from build123d import *

# Parameters (mm, degrees)
F1_DEPTH = 500
F2_R     = 33.415616


with BuildPart() as f1:
    # F0 (on Front) → F1 (new body, symmetric)
    with BuildSketch(Plane.XZ):
        Polygon((-141.84029, 131.140749), (-11.84029, 98.816335), (-11.84029, -98.816335), (-141.84029, -131.140749), (-141.84029, -249.530149), (236.54911, -249.530149), (236.54911, -131.140749), (106.54911, -98.816335), (106.54911, 98.816335), (236.54911, 131.140749), (236.54911, 249.530149), (-141.84029, 249.530149), align=None)
    extrude(amount=F1_DEPTH, both=True)

    # F2
    f2_edges = [f1.edges().sort_by_distance(p)[0] for p in [
        (106.54911, 0, -98.816335),
        (-11.84029, 0, 98.816335),
        (-11.84029, 0, -98.816335),
        (106.54911, 0, 98.816335),
    ]]
    fillet(f2_edges, radius=F2_R)


solid = f1.part
Work out the finished part from the listing and answer in its coordinate system (mm). A direction names the side the tool comes from. Give positions to 0.01 mm unless a question says otherwise; leave off trailing zeros. Write each loop counter-clockwise with the first axis right and the second up, starting at its lowest first coordinate (ties: lowest second). Pieces come first, ordered by that corner, then holes. Notation, with made-up numbers: (1.5, 40.5) - (32.5, 40.5) arc R12 cw to (32.5, 57.5) - close; hole circle Ø3 at (-31.75, 12.5). An arc over 180 degrees is marked (long way). One line per item, written item: value. Start each with the question number.
1. For a pull along Z with two mould halves and no side action, classify faces 4 (the flat face through (45, -500, 3)), 5 (the flat face through (50, -7, 249.53)), 6 (the flat face through (-89, -7, -118)), 7 (the cylindrical face through (113.832, -7, 93.517)) as +Z half, -Z half, draft (parallel to the pull), parting line (faces both ways), or undercut.
2. Find section A-A (x = -76.5). Write down the section's boundary in (y, z).
3. Given pin 1 (3 mm diameter, centred on y = -127.5, z = 89, fed in from -X); pin 2 (4 mm diameter, centred on y = 206.5, z = 66.5, fed in from -X); pin 3 (1 mm diameter, centred on y = -273, z = -84, fed in from +X), each flat-ended and moving along its own axis, determine where each tip first touches the part or whether it passes through.
4. Find section C-C (z = 63). Write down the section's boundary in (x, y), then the cut area to 3 significant figures.
5. Find section B-B (y = -295.5). Write down the section's boundary in (x, z).
6. Consider probe 1 along X at (y, z) = (346, -14); probe 2 along Z at (x, y) = (-52, -161); probe 3 along Z at (x, y) = (193.5, -86.5). Determine where each line is inside the solid, lowest interval first.
7. For faces 1 (the cylindrical face through (113.45, -7, -93.03)), 2 (the cylindrical face through (-19.123, -7, 93.517)), 3 (the flat face through (236.549, -7, 190)), determine the directions among +Z, -Z, +X, -X, +Y, -Y from which every point of the face is accessible in a straight line to the end or side of a thin tool.
Geometry results:
1. face 4: draft
1. face 5: +Z half
1. face 6: undercut
1. face 7: undercut
2. outline: (-500, -249.53) - (500, -249.53) - (500, -114.89) - (-500, -114.89) - close; (-500, 114.89) - (500, 114.89) - (500, 249.53) - (-500, 249.53) - close
3. pin 1: x = -16.98
3. pin 2: x = -11.84
3. pin 3: x = 108.7
4. outline: (-11.84, -500) - (106.55, -500) - (106.55, 500) - (-11.84, 500) - close
4. area: 118,000 mm2
5. outline: (-141.84, -249.53) - (236.55, -249.53) - (236.55, -131.14) - (131.9, -105.12) arc R33.42 cw to (106.55, -72.69) - (106.55, 72.69) arc R33.42 cw to (131.9, 105.12) - (236.55, 131.14) - (236.55, 249.53) - (-141.84, 249.53) - (-141.84, 131.14) - (-37.19, 105.12) arc R33.42 cw to (-11.84, 72.69) - (-11.84, -72.69) arc R33.42 cw to (-37.19, -105.12) - (-141.84, -131.14) - close
6. probe 1: -11.84 to 106.55
6. probe 2: -249.53 to -108.8, 108.8 to 249.53
6. probe 3: -249.53 to -120.44, 120.44 to 249.53
7. face 1: +X, +Y, -Y
7. face 2: -X, +Y, -Y
7. face 3: +Z, -Z, +X, +Y, -Y
